from build123d import *

# Parameters (mm, degrees)
BOSS_EXTRUDE1_DEPTH = 38.1
SKETCH2_R           = 7.9375
BOSS_EXTRUDE2_DEPTH = 31.75
BOSS_EXTRUDE3_START = 31.75
SKETCH3_R           = 7.9375
BOSS_EXTRUDE3_DEPTH = 31.75


with BuildPart() as part:
    # Sketch1 → Boss-Extrude1 (new body)
    with BuildSketch(Plane.XY):
        with BuildLine():
            Line((2.38125, 7.571892411), (2.38125, 9.953142411))
            Line((2.38125, 9.953142411), (-2.38125, 9.953142411))
            Line((-2.38125, 9.953142411), (-2.38125, 7.571892411))
            ThreePointArc((-2.38125, 7.571892411), (0, -7.9375), (2.38125, 7.571892411))
        make_face()
    extrude(amount=BOSS_EXTRUDE1_DEPTH)

    # Sketch2 → Boss-Extrude2 (add)
    with BuildSketch(Plane.XY.offset(38.1)):
        with Locations(Location((0, 0, 0), (0, 0, 107.457603124))):
            Circle(SKETCH2_R)
    extrude(amount=BOSS_EXTRUDE2_DEPTH)

    # Sketch3 → Boss-Extrude3 (add)
    with BuildSketch(Plane(origin=(0, 0, 0), x_dir=(-1, 0, 0), z_dir=(0, 0, -1)).offset(BOSS_EXTRUDE3_START)):
        Circle(SKETCH3_R)
    extrude(amount=-BOSS_EXTRUDE3_DEPTH)


solid = part.part
Geometry: final body of the model. Coordinates: model frame, mm. A direction names the side the tool comes from. Coordinates: 2 decimals unless noted, no trailing zeros. Loops run counter-clockwise (first coordinate to the right, second up) from the corner with the lowest first, then second, coordinate; pieces in that order, holes last. Notation, with made-up numbers: M 11,21 L 30,21 A9 ccw 30,30 Z; hole C 61,65 d1. An arc over 180 degrees is marked long. One line per item, written item: value. Start each with the question number.
1) Material intervals for L1, parallel to X at y = 9, z = 38; L2, parallel to Y at x = 7.25, z = 39; L3, parallel to Y at x = -3, z = 19, sorted ascending. Write a range as from..to.
2) Pin query (flat end, axial travel): P1, Ø5, axis at x = 4.5, z = -10, coming from the -Y side; P2, Ø0.7, axis at y = 8.5, z = 24, coming from the -X side; P3, Ø8, axis at y = 4, z = 49.5, coming from the -X side; P4, Ø4, axis at y = 4.5, z = 49.5, coming from the +X side. Return the tip coordinate at first contact, or that it passes through.
3) Cut plane C-C (y = -6). Return loops of the section in (x, z).
4) Cut plane A-A (x = 0). Return loops of the section in (y, z), then the cut area to 3 significant figures.
5) Reachability of faces 1 (the flat face through (-2.381, 9, 19)), 2 (the flat face through (0, 9.953, 19)), 3 (the flat face through (2.381, 9, 19)) from +Z, -Z, +X, -X, +Y, -Y: full face, straight path, thin tool, end or side. Return the list, or none.
6) Cut plane B-B (z = -15.5). Return loops of the section in (x, y) (1 decimal).
7) Cut plane D-D (z = 27). Return loops of the section in (x, y) (1 decimal).
Evaluation:
1. L1: -2.38..2.38
1. L2: -3.23..3.23
1. L3: -7.35..7.35
2. P1: y = -7.68
2. P2: x = -2.38
2. P3: x = -7.94
2. P4: x = 7.53
3. outline: M -5.2,-31.75 L 5.2,-31.75 L 5.2,69.85 L -5.2,69.85 Z
4. outline: M -7.94,-31.75 L 7.94,-31.75 L 7.94,0 L 9.95,0 L 9.95,38.1 L 7.94,38.1 L 7.94,69.85 L -7.94,69.85 Z
4. area: 1,690 mm^2
5. face 1: +Z, -Z, -X, +Y
5. face 2: +Z, -Z, +X, -X, +Y
5. face 3: +Z, -Z, +X, +Y
6. outline: C 0,0 d15.9
7. outline: M -2.4,7.6 A7.9 ccw long 2.4,7.6 L 2.4,10 L -2.4,10 Z
